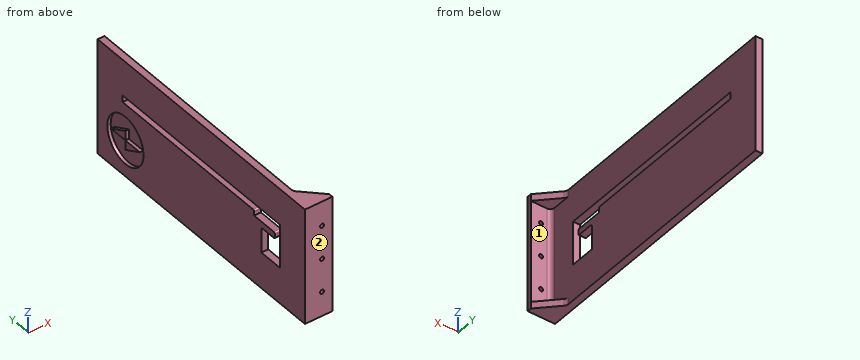
from build123d import *

# Parameters (mm, degrees)
SKETCH1_W               = 85
SKETCH1_H               = 200
BOSS_EXTRUDE1_DEPTH     = 5
FILLET1_R               = 1
SKETCH2_R               = 17.5
CUT_EXTRUDE1_DEPTH      = 2.5
FILLET2_R               = 0.125
SKETCH3_W               = 15
SKETCH3_H               = 85
BOSS_EXTRUDE2_DEPTH     = 3
RIB1_START              = -5
RIB1_DEPTH              = 5
SKETCH5_R               = 1.5
CUT_EXTRUDE2_DEPTH      = 3
FILLET3_R               = 4
FILLET4_R               = 3
MIRROR3_START           = -5
MIRROR3_COPY_1_DEPTH    = 5
FILLET5_R               = 4
FILLET6_R               = 3
CUT_EXTRUDE3_DEPTH      = 219.231528428
CUT_EXTRUDE3_DEPTH_BACK = 219.231528428
SKETCH7_R               = 17.5
BOSS_EXTRUDE3_DEPTH     = 2.5


# Read off the part's stored shape, not the designer's step: Rib1
with BuildPart() as part:
    # Sketch1 → Boss-Extrude1 (new body)
    with BuildSketch(Plane(origin=(0, 0, 0), x_dir=(0, 0, -1), z_dir=(1, 0, 0))):
        with Locations((0, 100)):
            Rectangle(SKETCH1_W, SKETCH1_H)
        Polygon((-16, 25), (-16, 176), (-11, 176), (-11, 49), (-7, 49), (-7, 29), (-2.5, 29), (-2.5, 42), (16, 42), (16, 25), (16, 24), (15, 24), (-15, 24), (-16, 24), align=None, mode=Mode.SUBTRACT)
    extrude(amount=BOSS_EXTRUDE1_DEPTH)

    # Fillet1
    fillet1_edges = [part.edges().sort_by_distance(p)[0] for p in [
        (2.5, 42, 2.5),
        (2.5, 29, 2.5),
        (2.5, 29, 7),
        (2.5, 49, 11),
    ]]
    fillet(fillet1_edges, radius=FILLET1_R)

    # Sketch2 → Cut-Extrude1 (cut)
    with BuildSketch(Plane(origin=(5, 0, 0), x_dir=(0, 0, -1), z_dir=(1, 0, 0))):
        with Locations((15.75, 173.25)):
            Circle(SKETCH2_R)
        Polygon((15.75, 173.125), (15.625, 173.25), (8.75, 173.25), (15.75, 187.25), (15.75, 173.375), (15.875, 173.25), (22.75, 173.25), (15.75, 159.25), align=None, mode=Mode.SUBTRACT)
    cut_extrude1 = extrude(amount=-CUT_EXTRUDE1_DEPTH, mode=Mode.SUBTRACT)

    # Fillet2
    fillet2_edges = [part.edges().sort_by_distance(p)[0] for p in [
        (3.75, 173.25, -15.625),
        (3.75, 173.125, -15.75),
        (3.75, 173.25, -15.875),
        (3.75, 173.375, -15.75),
    ]]
    fillet(fillet2_edges, radius=FILLET2_R)

    # Sketch3 → Boss-Extrude2 (add)
    with BuildSketch(Plane.XZ):
        with Locations((-7.5, 0)):
            Rectangle(SKETCH3_W, SKETCH3_H)
    boss_extrude2 = extrude(amount=-BOSS_EXTRUDE2_DEPTH)

    # Rib1 outline → Rib1 (add)
    with BuildSketch(Plane.XY.offset(42.5).offset(RIB1_START)):
        Polygon((0, 18), (-15, 3), (0, 3), align=None)
    rib1 = extrude(amount=RIB1_DEPTH)

    # Mirror1: Rib1 across plane
    add(rib1.mirror(Plane.XY))

    # Sketch5 → Cut-Extrude2 (cut)
    with BuildSketch(Plane(origin=(0, 3, 0), x_dir=(1, 0, 0), z_dir=(0, 1, 0))):
        with Locations(Location((-7.5, 24.5, 0), (0, 0, 270))):
            Circle(SKETCH5_R)
        with Locations(Location((-7.5, 0, 0), (0, 0, 270))):
            Circle(SKETCH5_R)
        with Locations(Location((-7.5, -24.5, 0), (0, 0, 270))):
            Circle(SKETCH5_R)
    cut_extrude2 = extrude(amount=-CUT_EXTRUDE2_DEPTH, mode=Mode.SUBTRACT)

    # Fillet3
    fillet3_edges = [part.edges().sort_by_distance(p)[0] for p in [
        (0, 18, 40),
        (0, 18, -40),
    ]]
    fillet(fillet3_edges, radius=FILLET3_R)

    # Fillet4
    fillet4_edges = [part.edges().sort_by_distance(p)[0] for p in [
        (0, 3, 0),
    ]]
    fillet(fillet4_edges, radius=FILLET4_R)

    # Mirror3: Boss-Extrude2, Rib1, Cut-Extrude2 across plane
    add(boss_extrude2.mirror(Plane(origin=(2.5, 0, 0), x_dir=(0, 0, 1), z_dir=(1, 0, 0))))
    add(rib1.mirror(Plane(origin=(2.5, 0, 0), x_dir=(0, 0, 1), z_dir=(1, 0, 0))))
    add(cut_extrude2.mirror(Plane(origin=(2.5, 0, 0), x_dir=(0, 0, 1), z_dir=(1, 0, 0))), mode=Mode.SUBTRACT)

    # Mirror3 copy 1 sketch → Mirror3 copy 1 (add)
    with BuildSketch(Plane(origin=(5, 0, -42.5), x_dir=(-1, 0, 0), z_dir=(0, 0, -1)).offset(MIRROR3_START)):
        Polygon((0, 18), (-15, 3), (0, 3), align=None)
    extrude(amount=MIRROR3_COPY_1_DEPTH)

    # Fillet5
    fillet5_edges = [part.edges().sort_by_distance(p)[0] for p in [
        (5, 18, 40),
        (5, 18, -40),
    ]]
    fillet(fillet5_edges, radius=FILLET5_R)

    # Fillet6
    fillet6_edges = [part.edges().sort_by_distance(p)[0] for p in [
        (5, 3, 0),
    ]]
    fillet(fillet6_edges, radius=FILLET6_R)

    # Sketch6 → Cut-Extrude3 (cut, two sides: drawn at the far end of the back side and taken through both)
    with BuildSketch(Plane.XY.offset(42.5).offset(-CUT_EXTRUDE3_DEPTH_BACK)):
        Polygon((0, 24), (0, -5.503420929), (-25.982696809, -6.518277055), (-24.822861237, 19.656854249), align=None)
    extrude(amount=CUT_EXTRUDE3_DEPTH + CUT_EXTRUDE3_DEPTH_BACK, mode=Mode.SUBTRACT)

    # Mirror4: Cut-Extrude1 across plane
    add(cut_extrude1.mirror(Plane(origin=(2.5, 0, 0), x_dir=(0, 0, 1), z_dir=(1, 0, 0))), mode=Mode.SUBTRACT)

    # Sketch7 → Boss-Extrude3 (add)
    with BuildSketch(Plane(origin=(5, 0, 0), x_dir=(0, 0, -1), z_dir=(1, 0, 0))):
        with Locations((15.75, 173.25)):
            Circle(SKETCH7_R)
    extrude(amount=-BOSS_EXTRUDE3_DEPTH)


solid = part.part
Design review of the part built by this model. Coordinates are the model's own, in mm. Face numbers are marked on the shaded views. A direction names the side the tool comes from. Round coordinates to 2 decimals unless told otherwise and drop trailing zeros. Order: outer loops, then holes, each group sorted by start corner. A loop starts at its lowest first (then second) coordinate and runs counter-clockwise, first axis right, second up.
1) Consider section B-B (z = -35). State the section outline as (x, y) points.
The answers:
outline: (0, 0) - (20, 0) - (20, 3) - (8, 3) arc R3 cw to (5, 6) - (5, 200) - (0, 200) - close
2) Consider section A-A (y = 54.5). State the section outline as (x, z) points, plus the area to 3 significant figures.
The answers:
outline: (0, -42.5) - (5, -42.5) - (5, 11) - (0, 11) - close; (0, 16) - (5, 16) - (5, 42.5) - (0, 42.5) - close
area: 400 mm2
3) Machinability: for the marked faces 1 and 2, which of the approach directions +Z, -Z, +X, -X, +Y, -Y give a long, thin tool a straight path to every point of the face, cutting with its end or side? Answer none if there is none.
The answers:
face 1: +X, +Y
face 2: +Z, -Z, +X, -X, -Y
4) For L1, parallel to Z at x = 12.5, y = 1.5; L2, parallel to Z at x = 3, y = 39.5; L3, parallel to Y at x = 1.75, z = 3.5, list the stretches that pass through material, from the lowest coordinate up.
The answers:
L1: z = -42.5 to -26, -23 to -1.5, 1.5 to 23, 26 to 42.5
L2: z = -42.5 to -16, 2.5 to 7, 16 to 42.5
L3: y = 0 to 24, 29 to 200
5) Clearance check with flat-ended pins moving along their axes: pin 1 Ø12 at (x, z) = (13.5, -28.5) entering from -Y; pin 2 Ø10 at (y, z) = (25.5, -21.5) entering from +X; pin 3 Ø3 at (x, z) = (12, 28) entering from +Y. State where each tip first meets the part, or that it passes through.
The answers:
pin 1: stops at y = 0
pin 2: stops at x = 5
pin 3: stops at y = 3
